Source: three-view drawing plus pictorial views. Frame: mm from the lowest corner of the part. Give positions to 0.01 mm unless a question says otherwise; leave off trailing zeros. Loops run counter-clockwise (first coordinate to the right, second up) from the corner with the lowest first, then second, coordinate; pieces in that order, holes last. Notation, with made-up numbers: M 89,-6.5 L 111,-6.5 A29 cw 111,28.5 Z; hole C 66.5,53 d6. An arc over 180 degrees is marked long. Write item = value, one per line.
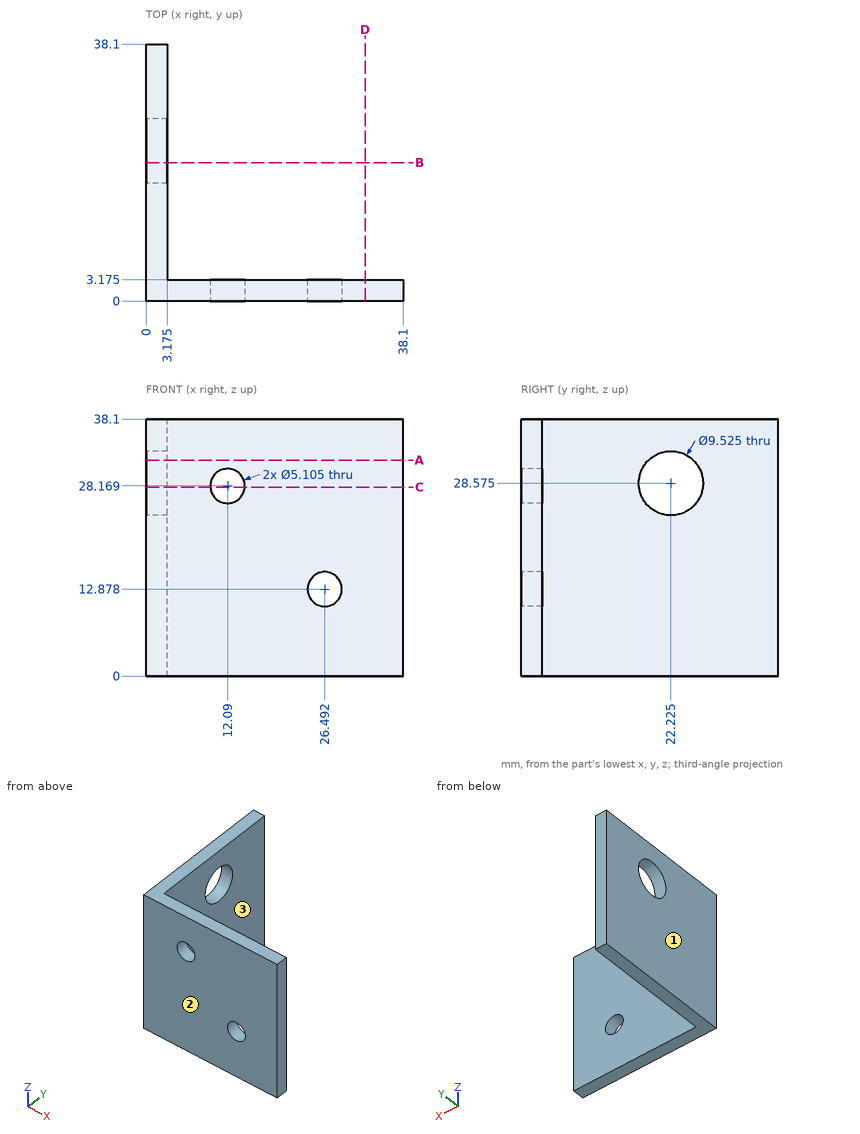
1. Cut plane B-B, the plane y = 20.5. Return the cut outline in (x, z) (1 decimal).
Derived:
outline = M 0,0 L 3.2,0 L 3.2,24.1 L 0,24.1 Z; M 0,33 L 3.2,33 L 3.2,38.1 L 0,38.1 Z
2. Cut plane D-D, the plane x = 32.5. Return the cut outline in (y, z) (1 decimal).
Derived:
outline = M 0,0 L 3.2,0 L 3.2,38.1 L 0,38.1 Z
3. Material intervals for probe 1 along Y at (x, z) = (11.5, 19) (1 decimal), sorted ascending. Write a range as from..to.
Derived:
probe_1 = 0..3.2
4. Pull-direction query (X, two-part tool) for the marked faces 1, 2 and 3; classes: +X half, -X half, draft (parallel to the pull), parting line (faces both ways), or undercut.
Derived:
face_1 = -X half
face_2 = draft
face_3 = +X half
5. Cut plane A-A, the plane z = 32. Return the cut outline in (x, y) (1 decimal).
Derived:
outline = M 0,0 L 38.1,0 L 38.1,3.2 L 3.2,3.2 L 3.2,18.9 L 0,18.9 Z; M 0,25.5 L 3.2,25.5 L 3.2,38.1 L 0,38.1 Z
6. First-contact query: pin 1 Ø6 at (x, z) = (12.09, 28.17) entering from -Y; pin 2 Ø17.5 at (y, z) = (20.5, 25.5) entering from +X (3 decimals); pin 3 Ø4 at (x, z) = (26.49, 12.88) entering from -Y; pin 4 Ø4 at (x, z) = (18, 7.5) entering from +Y (3 decimals). Flat tips, straight axial feed; report the tip coordinate or a pass-through.
Derived:
pin_1 = 0
pin_2 = 3.175
pin_3 = through
pin_4 = 3.175
7. Cut plane C-C, the plane z = 28. Return the cut outline in (x, y) (1 decimal), then the cut area to 3 significant figures.
Derived:
outline = M 0,0 L 9.5,0 L 9.5,3.2 L 3.2,3.2 L 3.2,17.5 L 0,17.5 Z; M 0,27 L 3.2,27 L 3.2,38.1 L 0,38.1 Z; M 14.6,0 L 38.1,0 L 38.1,3.2 L 14.6,3.2 Z
area = 186 mm²
